```python
from build123d import *

# Parameters (mm, degrees)
F0_W     = 203.2
F0_H     = 152.4
F1_DEPTH = 7.62
F2_W     = 13.762258
F2_H     = 14.236811
F3_DEPTH = 17.78


with BuildPart() as f1:
    # F0 (on Front) → F1 (new body)
    with BuildSketch(Plane.XZ):
        Rectangle(F0_W, F0_H)
    extrude(amount=F1_DEPTH)

    # F2 (on face) → F3 (join)
    with BuildSketch(Plane.XZ.offset(7.62)):
        with Locations((88.268232, 57.421802)):
            Rectangle(F2_W, F2_H)
        with Locations((88.268232, -57.421802)):
            Rectangle(F2_W, F2_H)
    extrude(amount=F3_DEPTH)


solid = f1.part
```
Geometry check sheet. Reference: the model listing, model coordinates, mm. A direction names the side the tool comes from. Give positions to 0.01 mm unless a question says otherwise; leave off trailing zeros. Write each loop counter-clockwise with the first axis right and the second up, starting at its lowest first coordinate (ties: lowest second). Pieces come first, ordered by that corner, then holes.
1) Section check D-D, the plane z = 14. Record the boundary of the cut face in (x, y).
2) Section check B-B, the plane z = 53. Record the boundary of the cut face in (x, y).
3) Section check A-A, the plane y = -12. Record the boundary of the cut face in (x, z), and give its area (3 significant figures).
4) Section check C-C, the plane x = -85.5. Record the boundary of the cut face in (y, z).
5) Gauge pin test, flat ends, axial feed: pin 1 (7 mm diameter, centred on y = -18, z = 60, fed in from +X); pin 2 (11 mm diameter, centred on x = 87, y = -17, fed in from -Z); pin 3 (7 mm diameter, centred on y = -17, z = -56, fed in from -X). Record the tip position at first contact, or that the pin passes through.
6) Release check for a two-part mould opening along Z. For faces 1 (the flat face through (88, -16, 50.303)), 2 (the flat face through (88, -25.4, 58)), 3 (the flat face through (-1, -4, 76.2)) record: pulls with the +Z half, pulls with the -Z half, needs draft (parallel to the pull), parting line crosses it, or undercut.
7) Material ranges on L1, parallel to Y at x = -4.5, z = 15.5; L2, parallel to X at y = -18.25, z = -60, recorded low to high.
8) Access from +Z, -Z, +X, -X, +Y, -Y to the whole of each face (thin tool, end or side, straight path). Record for faces 4 (the flat face through (88, -16, 64.54)), 5 (the flat face through (81.387, -16, 57)), 6 (the flat face through (95.149, -16, 57)).
Computed:
1. outline: (-101.6, -7.62) - (101.6, -7.62) - (101.6, 0) - (-101.6, 0) - close
2. outline: (-101.6, -7.62) - (81.39, -7.62) - (81.39, -25.4) - (95.15, -25.4) - (95.15, -7.62) - (101.6, -7.62) - (101.6, 0) - (-101.6, 0) - close
3. outline: (81.39, -64.54) - (95.15, -64.54) - (95.15, -50.3) - (81.39, -50.3) - close; (81.39, 50.3) - (95.15, 50.3) - (95.15, 64.54) - (81.39, 64.54) - close
3. area: 392 mm2
4. outline: (-7.62, -76.2) - (0, -76.2) - (0, 76.2) - (-7.62, 76.2) - close
5. pin 1: stops at x = 95.15
5. pin 2: stops at z = -64.54
5. pin 3: stops at x = 81.39
6. face 1: undercut
6. face 2: needs draft
6. face 3: pulls with the +Z half
7. L1: y = -7.62 to 0
7. L2: x = 81.39 to 95.15
8. face 4: +Z, +X, -X, -Y
8. face 5: +Z, -Z, -X, -Y
8. face 6: +Z, -Z, +X, -Y
